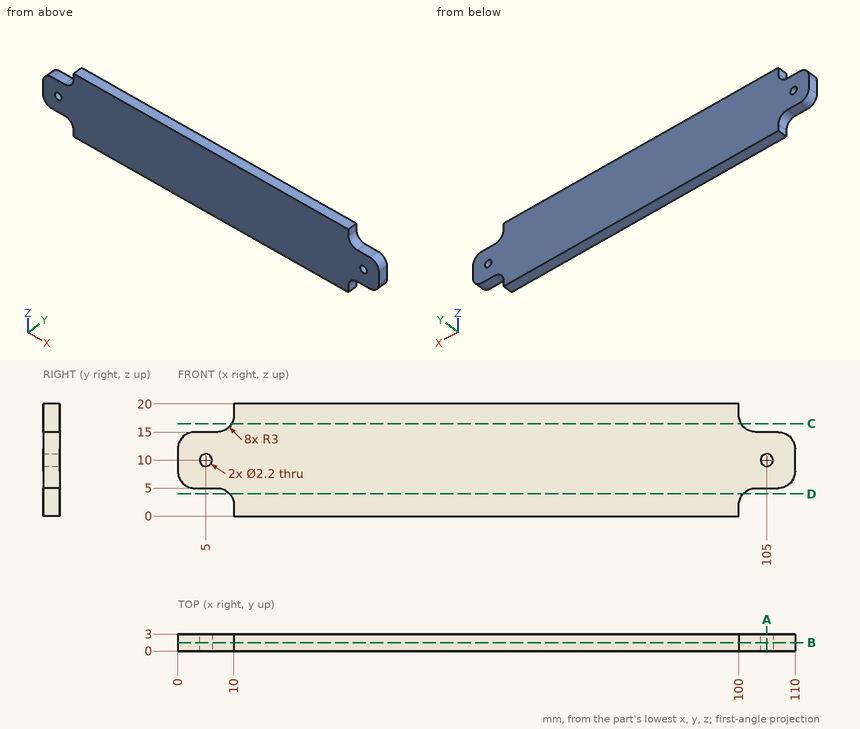
For this review, use the dimensioned drawing (mm, ordinates from the lowest corner) and the shaded views. Coordinates: 2 decimals unless noted, no trailing zeros. Order: outer loops, then holes, each group sorted by start corner. A loop starts at its lowest first (then second) coordinate and runs counter-clockwise, first axis right, second up. Notation, with made-up numbers: M 52,2 L 69,2 A26 ccw 69,24 Z; hole C 52,50 d11. An arc over 180 degrees is marked long. Answer as a JSON object with one key per item and string values. Group by question number.
1) Add section C-C, the plane z = 16.5. Write out the cut boundary in (x, y), then the cut area to 3 significant figures.
2) Add section D-D, the plane z = 4. Write out the cut boundary in (x, y).
3) Add section B-B, the plane y = 1.5. Write out the cut boundary in (x, z).
4) For pin 1 (1.5 mm diameter, centred on y = 1, z = 3.5, fed in from -X); pin 2 (0.6 mm diameter, centred on y = 1, z = 1, fed in from -X); pin 3 (1 mm diameter, centred on y = 0.5, z = 16, fed in from +X), all flat-tipped, find the tip position at first contact; note any pin that passes through.
5) Wall thickness on L1, parallel to Z at x = 105, y = 2; L2, parallel to X at y = 2.7, z = 9.25; L3, parallel to X at y = 2.5, z = 11: over which ranges is each line inside the solid? List them lowest first.
6) Add section A-A, the plane x = 105. Write out the cut boundary in (y, z), then the cut area to 3 significant figures.
Computed values:
{
 "1": {"outline": "M 9.6,0 L 100.4,0 L 100.4,3 L 9.6,3 Z", "area": "272 mm^2"},
 "2": {"outline": "M 9.24,0 L 100.76,0 L 100.76,3 L 9.24,3 Z"},
 "3": {"outline": "M 0,8 A3 ccw 3,5 L 7,5 A3 cw 10,2 L 10,0 L 100,0 L 100,2 A3 cw 103,5 L 107,5 A3 ccw 110,8 L 110,12 A3 ccw 107,15 L 103,15 A3 cw 100,18 L 100,20 L 10,20 L 10,18 A3 cw 7,15 L 3,15 A3 ccw 0,12 Z; hole C 5,10 d2.2; hole C 105,10 d2.2"},
 "4": {"pin 1": "stops at x = 8.98", "pin 2": "stops at x = 10", "pin 3": "stops at x = 101.34"},
 "5": {"L1": "z = 5 to 8.9, 11.1 to 15", "L2": "x = 0 to 4.2, 5.8 to 104.2, 105.8 to 110", "L3": "x = 0 to 4.54, 5.46 to 104.54, 105.46 to 110"},
 "6": {"outline": "M 0,5 L 3,5 L 3,8.9 L 0,8.9 Z; M 0,11.1 L 3,11.1 L 3,15 L 0,15 Z", "area": "23.4 mm^2"}
}
